```python
from build123d import *

# Parameters (mm, degrees)
F0_W     = 250
F0_H     = 170
F0_W_2   = 235
F0_H_2   = 150
F1_DEPTH = 3
F2_W     = 250
F2_H     = 170
F2_W_2   = 225
F2_H_2   = 135
F3_DEPTH = 82
F4_R     = 10


with BuildPart() as f1:
    # F0 (on Top) → F1 (new body)
    with BuildSketch(Plane.XY):
        Rectangle(F0_W, F0_H)
        Rectangle(F0_W_2, F0_H_2, mode=Mode.SUBTRACT)
        Rectangle(F0_W_2, F0_H_2)
    extrude(amount=F1_DEPTH)

    # F2 (on face) → F3 (join)
    with BuildSketch(Plane.XY.offset(3)):
        Rectangle(F2_W, F2_H)
        Rectangle(F2_W_2, F2_H_2, mode=Mode.SUBTRACT)
    extrude(amount=-F3_DEPTH)

    # F4
    f4_edges = [f1.edges().sort_by_distance(p)[0] for p in [
        (-125, 0, 3),
        (0, -85, 3),
        (125, 0, 3),
        (0, 85, 3),
        (125, -85, -38),
        (125, 85, -38),
        (-125, -85, -38),
        (-125, 85, -38),
    ]]
    fillet(f4_edges, radius=F4_R)


solid = f1.part
```
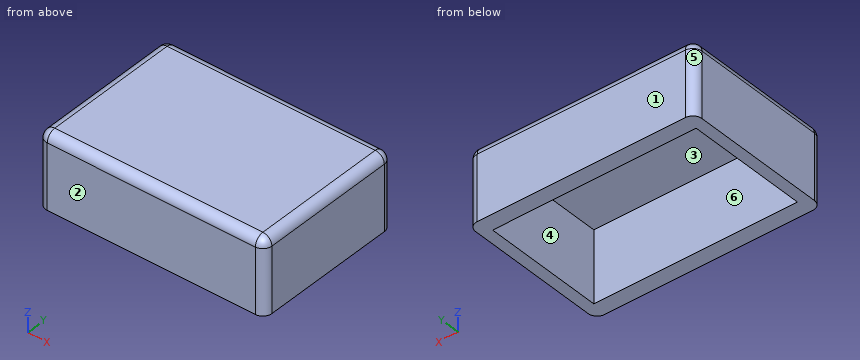
The model under review builds one solid part; all positions refer to its coordinate system, in mm. Face numbers are marked on the shaded views. A direction names the side the tool comes from. Give positions to 0.01 mm unless a question says otherwise; leave off trailing zeros. Write each loop counter-clockwise with the first axis right and the second up, starting at its lowest first coordinate (ties: lowest second). Pieces come first, ordered by that corner, then holes. Notation, with made-up numbers: M 35,87.5 L 94,87.5 A12 ccw 94,101.5 Z; hole C -35.5,29.5 d8. An arc over 180 degrees is marked long. Answer in a Markdown table with one row per item.
Item 1: Add section C-C on y = 22. Give the boundary of the cut face in (x, z), plus the area to 3 significant figures.
Check sheet entries:
| item | result |
|---|---|
| outline | M -125,-79 L -112.5,-79 L -112.5,0 L 112.5,0 L 112.5,-79 L 125,-79 L 125,-7 A10 ccw 115,3 L -115,3 A10 ccw -125,-7 Z |
| area | 2,680 mm2 |
Item 2: Tool access review of the marked faces 5 and 6: name each direction out of +Z, -Z, +X, -X, +Y, -Y from which nothing blocks a thin tool from reaching the whole face with its end or side.
Check sheet entries:
| item | result |
|---|---|
| face 5 | +Z, -Z, -X, +Y |
| face 6 | -Z |
Item 3: For P1, Ø10, axis at x = -44.5, y = -2.5, coming from the -Z side, flat-tipped, find the tip position at first contact; note if it passes through.
Check sheet entries:
| item | result |
|---|---|
| P1 | z = 0 |
Item 4: For line 1 along Y through (x, z) = (89.5, -39); line 2 along X through (y, z) = (23, -25); line 3 along Z through (x, y) = (41.5, 31), list the stretches that pass through material, from the lowest coordinate up.
Check sheet entries:
| item | result |
|---|---|
| line 1 | -85 to -67.5, 67.5 to 85 |
| line 2 | -125 to -112.5, 112.5 to 125 |
| line 3 | 0 to 3 |
Item 5: Add section A-A on z = -68. Give the boundary of the cut face in (x, y), plus the area to 3 significant figures.
Check sheet entries:
| item | result |
|---|---|
| outline | M -125,-75 A10 ccw -115,-85 L 115,-85 A10 ccw 125,-75 L 125,75 A10 ccw 115,85 L -115,85 A10 ccw -125,75 Z; hole M -112.5,-67.5 L 112.5,-67.5 L 112.5,67.5 L -112.5,67.5 Z |
| area | 12,000 mm2 |
Item 6: Draft analysis for pull direction Y (two halves, no side actions). For the marked faces 1, 2, 3 and 4, state which applies: +Y half, -Y half, draft (parallel to the pull), parting line (faces both ways), or undercut.
Check sheet entries:
| item | result |
|---|---|
| face 1 | +Y half |
| face 2 | -Y half |
| face 3 | undercut |
| face 4 | undercut |
Item 7: Add section B-B on x = 90.5. Give the boundary of the cut face in (y, z).
Check sheet entries:
| item | result |
|---|---|
| outline | M -85,-79 L -67.5,-79 L -67.5,0 L 67.5,0 L 67.5,-79 L 85,-79 L 85,-7 A10 ccw 75,3 L -75,3 A10 ccw -85,-7 Z |
